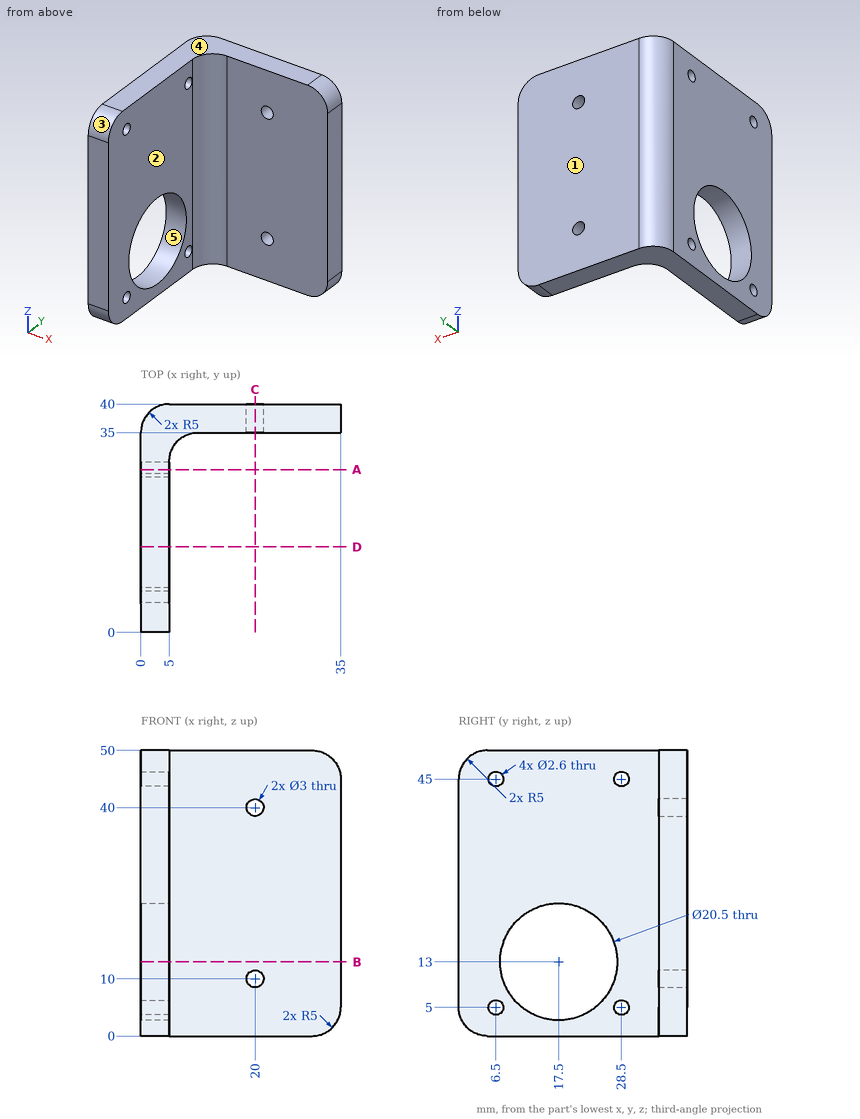
Source: three-view drawing plus pictorial views. Frame: mm from the lowest corner of the part. A direction names the side the tool comes from. Give positions to 0.01 mm unless a question says otherwise; leave off trailing zeros. Order: outer loops, then holes, each group sorted by start corner. A loop starts at its lowest first (then second) coordinate and runs counter-clockwise, first axis right, second up. Notation, with made-up numbers: M -37,68.25 L -33,68.25 A12 ccw -33,83.25 Z; hole C 29,34 d10. An arc over 180 degrees is marked long. One line per question, with ' | ' between items. Start each with the question number.
1. Section query D-D (y = 15). Return the cut outline in (x, z), and give its area (3 significant figures).
2. Material intervals for probe 1 along Y at (x, z) = (2, 5); probe 2 along Y at (x, z) = (3, 45); probe 3 along Y at (x, z) = (3.75, 45), sorted ascending. Write a range as [from, to].
3. Section query A-A (y = 28.5). Return the cut outline in (x, z).
4. Access query for the marked faces 1 and 2. Directions: +Z, -Z, +X, -X, +Y, -Y. A direction counts if a zero-diameter tool reaches every point of the face in a straight line with its end or side. Return the directions, or none.
5. First-contact query: pin 1 Ø4 at (y, z) = (28.5, 5) entering from +X; pin 2 Ø7.5 at (x, z) = (27.5, 21.5) entering from -Y. Flat tips, straight axial feed; report the tip coordinate or a pass-through.
6. Section query B-B (z = 13). Return the cut outline in (x, y).
7. Pull-direction query (Y, two-part tool) for the marked faces 3, 4 and 5; classes: released by +Y, released by -Y, zero draft, split by the parting line, or undercut.
8. Section query C-C (x = 20). Return the cut outline in (y, z), and give its area (3 significant figures).
Here are the results:
1) outline: M 0,0 L 5,0 L 5,3.06 L 0,3.06 Z; M 0,22.94 L 5,22.94 L 5,50 L 0,50 Z | area: 151 mm²
2) probe 1: [0, 5.2], [7.8, 11.09], [23.91, 27.2], [29.8, 39] | probe 2: [0, 5.2], [7.8, 27.2], [29.8, 39.58] | probe 3: [0, 5.2], [7.8, 27.2], [29.8, 39.84]
3) outline: M 0,0 L 5,0 L 5,3.7 L 0,3.7 Z; M 0,6.3 L 5,6.3 L 5,43.7 L 0,43.7 Z; M 0,46.3 L 5,46.3 L 5,50 L 0,50 Z
4) face 1: +Z, -Z, +X, -X, +Y | face 2: +Z, -Z, +X, -Y
5) pin 1: x = 5.03 | pin 2: y = 35
6) outline: M 0,0 L 5,0 L 5,7.25 L 0,7.25 Z; M 0,27.75 L 5,27.75 L 5,30 A5 cw 10,35 L 35,35 L 35,40 L 5,40 A5 ccw 0,35 Z
7) face 3: released by -Y | face 4: zero draft | face 5: undercut
8) outline: M 35,0 L 40,0 L 40,8.5 L 35,8.5 Z; M 35,11.5 L 40,11.5 L 40,38.5 L 35,38.5 Z; M 35,41.5 L 40,41.5 L 40,50 L 35,50 Z | area: 220 mm²
